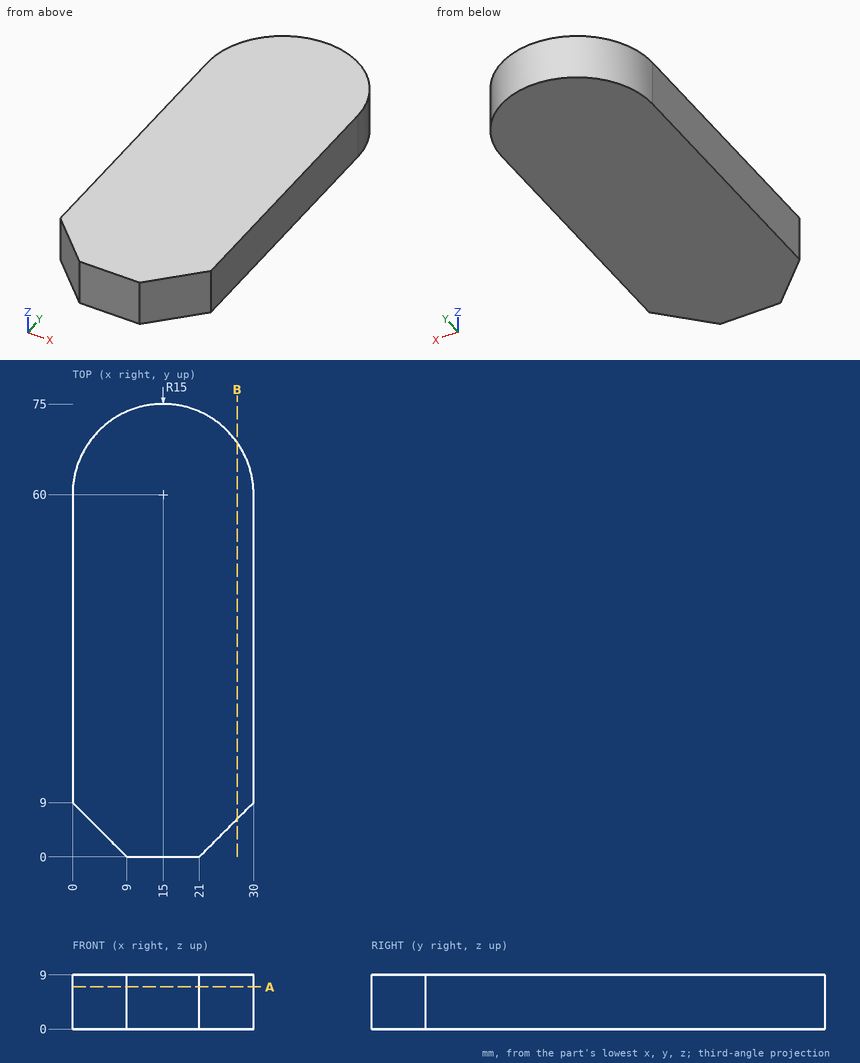
Study the drawing (mm; zero at the part's minimum x, y, z) and answer. Give positions to 0.01 mm unless a question says otherwise; leave off trailing zeros. Loops run counter-clockwise (first coordinate to the right, second up) from the corner with the lowest first, then second, coordinate; pieces in that order, holes last. Notation, with made-up numbers: (4, 66.25) -> (25, 66.25) arc R6 cw to (25, 74.25) -> close; hole circle Ø7 at (-19.75, 88). An arc over 180 degrees is marked (long way). Write item = value, one per line. Start each with the question number.
(1) Find section A-A on z = 7. Give the vertices of the cut face in (x, y), and give its area (3 significant figures).
(2) Find the intervals of material crossed by probe 1 along Y at (x, z) = (15.25, 7.75); probe 2 along Y at (x, z) = (19.5, 3.25); probe 3 along X at (y, z) = (68, 2), in increasing order. Write a range as from..to.
(3) Find section B-B on x = 27.25. Give the vertices of the cut face in (y, z).
From the geometry:
q1.outline = (0, 9) -> (9, 0) -> (21, 0) -> (30, 9) -> (30, 60) arc R15 ccw to (0, 60) -> close
q1.area = 2,070 mm^2
q2.probe_1 = 0..75
q2.probe_2 = 0..74.31
q2.probe_3 = 2.31..27.69
q3.outline = (6.25, 0) -> (68.66, 0) -> (68.66, 9) -> (6.25, 9) -> close
